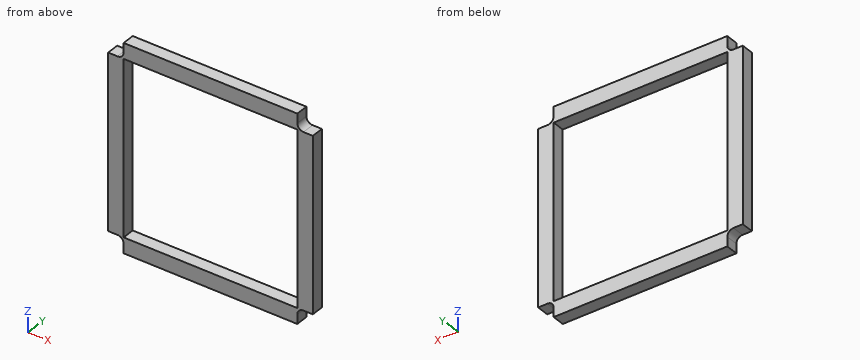
from build123d import *

# Parameters (mm, degrees)
CROQUIS1_W              = 165
CROQUIS1_H              = 165
CROQUIS1_W_2            = 140
CROQUIS1_H_2            = 140
SALIENTE_EXTRUIR1_DEPTH = 10
CORTAR_EXTRUIR1_DEPTH   = 10


with BuildPart() as part:
    # Croquis1 → Saliente-Extruir1 (new body)
    with BuildSketch(Plane(origin=(0, 0, 0), x_dir=(1, 0, 0), z_dir=(0, 1, 0))):
        with Locations((70, 70)):
            Rectangle(CROQUIS1_W, CROQUIS1_H)
        with Locations((70, 70)):
            Rectangle(CROQUIS1_W_2, CROQUIS1_H_2, mode=Mode.SUBTRACT)
    extrude(amount=SALIENTE_EXTRUIR1_DEPTH)

    # Croquis2 → Cortar-Extruir1 (cut)
    with BuildSketch(Plane(origin=(0, 10, 0), x_dir=(1, 0, 0), z_dir=(0, 1, 0))):
        with BuildLine():
            Line((0, 145), (0, 152.5))
            Line((0, 152.5), (-12.5, 152.5))
            Line((-12.5, 152.5), (-12.5, 140))
            Line((-12.5, 140), (-5, 140))
            ThreePointArc((-5, 140), (-1.464466094, 141.464466094), (0, 145))
        make_face()
        with BuildLine():
            Line((145, 140), (152.5, 140))
            Line((152.5, 140), (152.5, 152.5))
            Line((152.5, 152.5), (140, 152.5))
            Line((140, 152.5), (140, 145))
            ThreePointArc((140, 145), (141.464466094, 141.464466094), (145, 140))
        make_face()
        with BuildLine():
            Line((140, -5), (140, -12.5))
            Line((140, -12.5), (152.5, -12.5))
            Line((152.5, -12.5), (152.5, 0))
            Line((152.5, 0), (145, 0))
            ThreePointArc((145, 0), (141.464466094, -1.464466094), (140, -5))
        make_face()
        with BuildLine():
            Line((-5, 0), (-12.5, 0))
            Line((-12.5, 0), (-12.5, -12.5))
            Line((-12.5, -12.5), (0, -12.5))
            Line((0, -12.5), (0, -5))
            ThreePointArc((0, -5), (-1.464466094, -1.464466094), (-5, 0))
        make_face()
    extrude(amount=-CORTAR_EXTRUIR1_DEPTH, mode=Mode.SUBTRACT)


solid = part.part
Can you work these out from the model? Positions are in its coordinate system, mm. Round coordinates to 2 decimals unless told otherwise and drop trailing zeros. Write each loop counter-clockwise with the first axis right and the second up, starting at its lowest first coordinate (ties: lowest second). Pieces come first, ordered by that corner, then holes. Notation, with made-up numbers: (-5.75, 23.5) -> (1.25, 23.5) arc R13 ccw to (1.25, 44.5) -> close; hole circle Ø7 at (59, 43.25). An arc over 180 degrees is marked (long way). One line per question, with ' | ' between items. Start each with the question number.
1) Suppose I cut it at C-C on x = 93.5. Write out the boundary of the cut face in (y, z), then the cut area to 3 significant figures.
2) Suppose I cut it at B-B on y = 4.75. Write out the boundary of the cut face in (x, z), then the cut area to 3 significant figures.
3) Suppose I cut it at A-A on z = -73. Write out the boundary of the cut face in (x, y), then the cut area to 3 significant figures.
4) I need wall thicknesses on line 1 (X direction, y = 8, z = -130); line 2 (Z direction, x = 1, y = 2.25); line 3 (X direction, y = 8.25, z = 2.5). Which ranges of each line are inside material? Lowest first, please. Write a range as [from, to].
5) I'm going to push flat-ended pins straight in: P1, Ø6, axis at x = 148.5, y = 3, coming from the +Z side; P2, Ø4, axis at y = 4, z = -149, coming from the +X side; P3, Ø4, axis at y = 3.5, z = -148, coming from the -X side. Where does each tip first touch, or does it pass through?
Return value:
1) outline: (0, -152.5) -> (10, -152.5) -> (10, -140) -> (0, -140) -> close; (0, 0) -> (10, 0) -> (10, 12.5) -> (0, 12.5) -> close | area: 250 mm2
2) outline: (-12.5, -140) -> (-5, -140) arc R5 cw to (0, -145) -> (0, -152.5) -> (140, -152.5) -> (140, -145) arc R5 cw to (145, -140) -> (152.5, -140) -> (152.5, 0) -> (145, 0) arc R5 cw to (140, 5) -> (140, 12.5) -> (0, 12.5) -> (0, 5) arc R5 cw to (-5, 0) -> (-12.5, 0) -> close; hole (0, -140) -> (140, -140) -> (140, 0) -> (0, 0) -> close | area: 7,020 mm2
3) outline: (-12.5, 0) -> (0, 0) -> (0, 10) -> (-12.5, 10) -> close; (140, 0) -> (152.5, 0) -> (152.5, 10) -> (140, 10) -> close | area: 250 mm2
4) line 1: x = [-12.5, 0], [140, 152.5] | line 2: z = [-152.5, -140], [0, 12.5] | line 3: x = [-0.67, 140.67]
5) P1: stops at z = 0 | P2: stops at x = 140 | P3: stops at x = 0
